```python
from build123d import *

# Parameters (mm, degrees)
SKETCH_1_W        = 13
SKETCH_1_H        = 6.5
SKETCH_1_R        = 1
EXTRUDE_1_DEPTH   = 3
SKETCH_2_R        = 0.5
EXTRUDE_2_DEPTH   = 4
EXTRUDE_1_2_DEPTH = 2


with BuildPart() as part:
    # Эскиз1 → Extrude 1 (new, symmetric)
    with BuildSketch(Plane(origin=(0, 0, 0), x_dir=(1, 0, 0), z_dir=(0, 1, 0))):
        Rectangle(SKETCH_1_W, SKETCH_1_H)
        with Locations(Location((3.25, -1.75, 0), (0, 0, 270))):
            Circle(SKETCH_1_R, mode=Mode.SUBTRACT)
        with Locations(Location((-3.25, -1.75, 0), (0, 0, 90))):
            Circle(SKETCH_1_R, mode=Mode.SUBTRACT)
    extrude(amount=EXTRUDE_1_DEPTH, both=True)

    # Эскиз2 → Бобышка-Вытянуть2 (add)
    with BuildSketch(Plane.XY.offset(3.25)):
        with Locations(Location((-3.264227948, 0, 0), (0, 0, 180))):
            Circle(SKETCH_2_R)
        with Locations(Location((0, 0, 0), (0, 0, 180))):
            Circle(SKETCH_2_R)
        with Locations(Location((3.264227948, 0, 0), (0, 0, 180))):
            Circle(SKETCH_2_R)
    extrude(amount=EXTRUDE_2_DEPTH)

    # Эскиз3 → Extrude 1 2 (add, symmetric)
    with BuildSketch(Plane(origin=(0, 0, 0), x_dir=(1, 0, 0), z_dir=(0, 1, 0))):
        Polygon((-6.471609365, 3.1282668), (7.594638597, 6.4087992), (7.537857328, 6.6522656), (-6.528390635, 3.3717332), align=None)
    extrude(amount=EXTRUDE_1_2_DEPTH, both=True)


solid = part.part
```
Geometry check sheet. Reference: the model listing, model coordinates, mm. A direction names the side the tool comes from. Coordinates: 2 decimals unless noted, no trailing zeros. Loops run counter-clockwise (first coordinate to the right, second up) from the corner with the lowest first, then second, coordinate; pieces in that order, holes last. Notation, with made-up numbers: (-37, 86.25) -> (-28, 86.25) arc R8 cw to (-28, 92.25) -> close; hole circle Ø9 at (58.5, -11.75). An arc over 180 degrees is marked (long way). Put each result on its own line as item: value.
1) Gauge pin test, flat ends, axial feed: pin 1 Ø1.7 at (x, z) = (1.5, -4.5) entering from +Y; pin 2 Ø3 at (x, z) = (-3.25, 1.75) entering from +Y; pin 3 Ø1.8 at (y, z) = (0.5, 0.5) entering from +X; pin 4 Ø2 at (x, y) = (2.5, 2) entering from +Z. Record the tip position at first contact, or that the pin passes through.
Result set:
pin 1: stops at y = 2
pin 2: stops at y = 3
pin 3: stops at x = 6.5
pin 4: stops at z = 3.25
2) Cross-section at C-C on x = 0. Record the boundary of the cut face in (y, z).
Result set:
outline: (-3, -3.25) -> (3, -3.25) -> (3, 3.25) -> (0.5, 3.25) -> (0.5, 7.25) -> (-0.5, 7.25) -> (-0.5, 3.25) -> (-3, 3.25) -> close; (-2, -4.89) -> (2, -4.89) -> (2, -4.64) -> (-2, -4.64) -> close
3) Thickness scan on line 1 (X direction, y = -1.3, z = 1.75); line 2 (Z direction, x = -3.25, y = 1); line 3 (Z direction, x = -3.25, y = -0.05). Record the ranges inside material, lowest first.
Result set:
line 1: x = -6.5 to -4.25, -2.25 to 2.25, 4.25 to 6.5
line 2: z = -4.14 to -3.88, -3.25 to 0.75, 2.75 to 3.25
line 3: z = -4.14 to -3.88, -3.25 to 0.75, 2.75 to 7.25
4) Tool access check on faces 5 (the cylindrical face through (2.8, 0.19, 5.22)), 6 (the flat face through (0.7, 0, -4.8)), 7 (the flat face through (0, -3, 0)), 8 (the flat face through (6.5, 0, 0)). Record the directions out of +Z, -Z, +X, -X, +Y, -Y that give a thin tool (end or side, any length) a straight path to the whole face; none if there is none.
Result set:
face 5: +Z
face 6: +X, +Y, -Y
face 7: +Z, -Z, +X, -X, -Y
face 8: +Z, +X, +Y, -Y
5) Release check for a two-part mould opening along Z. For faces 1 (the flat face through (0.603, 0.028, -5.035)), 2 (the flat face through (-6.5, 0, 0)), 3 (the flat face through (0, 0, -3.25)), 4 (the cylindrical face through (4.24, -0.04, 1.62)) record: released by +Z, released by -Z, zero draft, split by the parting line, or undercut.
Result set:
face 1: released by -Z
face 2: zero draft
face 3: undercut
face 4: undercut
6) Cross-section at B-B on y = 0. Record the boundary of the cut face in (x, z), plus the area to 3 significant figures.
Result set:
outline: (-6.53, -3.37) -> (7.54, -6.65) -> (7.59, -6.41) -> (-5.95, -3.25) -> (6.5, -3.25) -> (6.5, 3.25) -> (3.76, 3.25) -> (3.76, 7.25) -> (2.76, 7.25) -> (2.76, 3.25) -> (0.5, 3.25) -> (0.5, 7.25) -> (-0.5, 7.25) -> (-0.5, 3.25) -> (-2.76, 3.25) -> (-2.76, 7.25) -> (-3.76, 7.25) -> (-3.76, 3.25) -> (-6.5, 3.25) -> (-6.5, -3.25) -> close; hole circle Ø2 at (-3.25, 1.75); hole circle Ø2 at (3.25, 1.75)
area: 93.8 mm^2
7) Cross-section at D-D on x = -3.5. Record the boundary of the cut face in (y, z), plus the area to 3 significant figures.
Result set:
outline: (-3, -3.25) -> (3, -3.25) -> (3, 0.78) -> (-3, 0.78) -> close; (-3, 2.72) -> (3, 2.72) -> (3, 3.25) -> (0.44, 3.25) -> (0.44, 7.25) -> (-0.44, 7.25) -> (-0.44, 3.25) -> (-3, 3.25) -> close; (-2, -4.08) -> (2, -4.08) -> (2, -3.82) -> (-2, -3.82) -> close
area: 31.9 mm^2
8) Cross-section at A-A on z = 1.75. Record the boundary of the cut face in (x, y).
Result set:
outline: (-6.5, -3) -> (-4.25, -3) -> (-4.25, 3) -> (-6.5, 3) -> close; (-2.25, -3) -> (2.25, -3) -> (2.25, 3) -> (-2.25, 3) -> close; (4.25, -3) -> (6.5, -3) -> (6.5, 3) -> (4.25, 3) -> close
